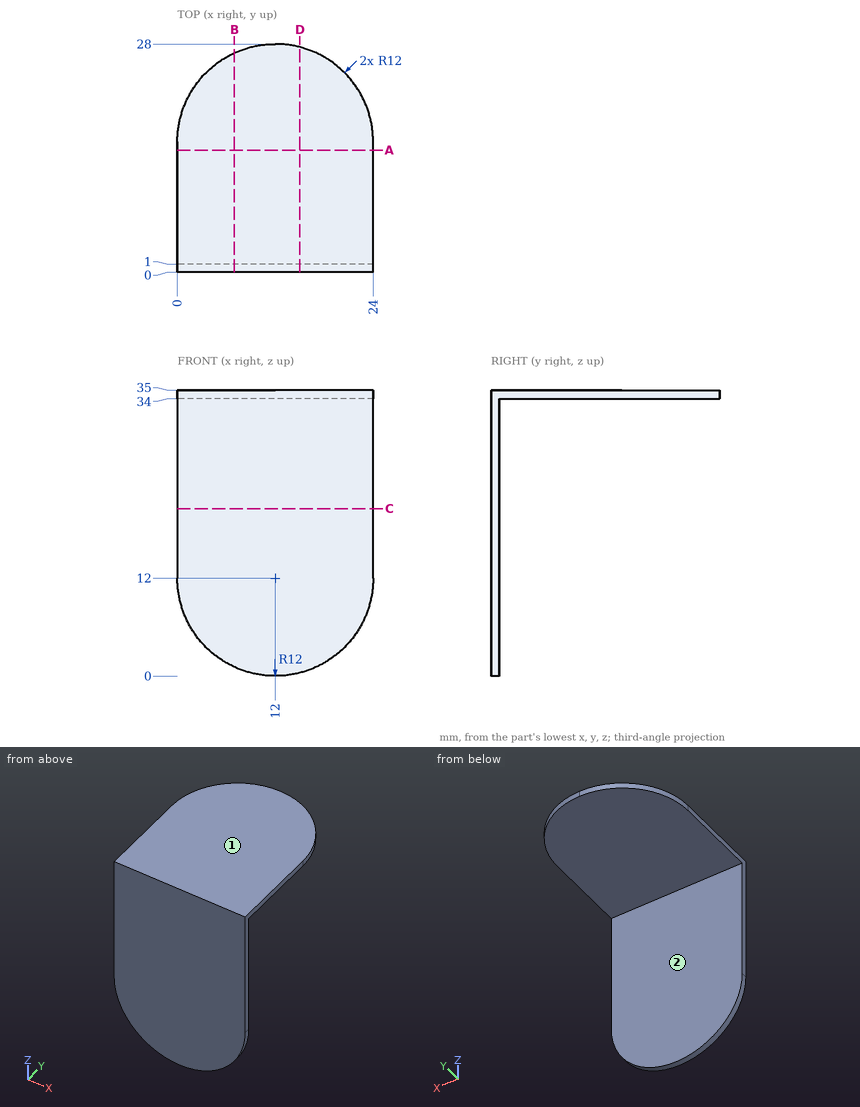
Here's the drawing with two shaded views (mm, measured from the low corner). I have some questions. A direction names the side the tool comes from. Give positions to 0.01 mm unless a question says otherwise; leave off trailing zeros. Write each loop counter-clockwise with the first axis right and the second up, starting at its lowest first coordinate (ties: lowest second). Pieces come first, ordered by that corner, then holes. Notation, with made-up numbers: (-2.75, -16) - (20.25, -16) arc R22 cw to (20.25, -8) - close; hole circle Ø6 at (22, 7.5). An arc over 180 degrees is marked (long way). Write item = value, one per line. Start each with the question number.
1. For pin 1 (12 mm diameter, centred on y = 24.5, z = 27.5, fed in from -X); pin 2 (3 mm diameter, centred on x = 9.5, z = 18, fed in from +Y), each with a flat end and sliding along its axis, tell me the tip position at first contact or that it passes through.
2. Imagine slicing it at B-B (x = 7). Please give me the cut outline in (y, z), and give its area (3 significant figures).
3. Please list where these lines run through material, in increasing order: line 1 (Y direction, x = 16, z = 20); line 2 (Z direction, x = 23.25, y = 14.75).
4. Imagine slicing it at A-A (y = 15). Please give me the cut outline in (x, z), and give its area (3 significant figures).
5. Imagine slicing it at D-D (x = 15). Please give me the cut outline in (y, z).
6. On a 3-axis mill with a long thin cutter (end or side, diameter ignored), from which of +Z, -Z, +X, -X, +Y, -Y can I reach the whole of each face in a straight line? I mean the marked faces 1 and 2. Say none if no direction works.
7. Imagine slicing it at C-C (z = 20.5). Please give me the cut outline in (x, y), and give its area (3 significant figures).
Worked answers:
q1.pin_1 = through
q1.pin_2 = 1
q2.outline = (0, 1.09) - (1, 1.09) - (1, 34) - (26.91, 34) - (26.91, 35) - (0, 35) - close
q2.area = 59.8 mm2
q3.line_1 = 0 to 1
q3.line_2 = 34 to 35
q4.outline = (0, 34) - (24, 34) - (24, 35) - (0, 35) - close
q4.area = 24.0 mm2
q5.outline = (0, 0.38) - (1, 0.38) - (1, 34) - (27.62, 34) - (27.62, 35) - (0, 35) - close
q6.face_1 = +Z, +X, -X, +Y, -Y
q6.face_2 = -Z, +X, -X, +Y
q7.outline = (0, 0) - (24, 0) - (24, 1) - (0, 1) - close
q7.area = 24.0 mm2
